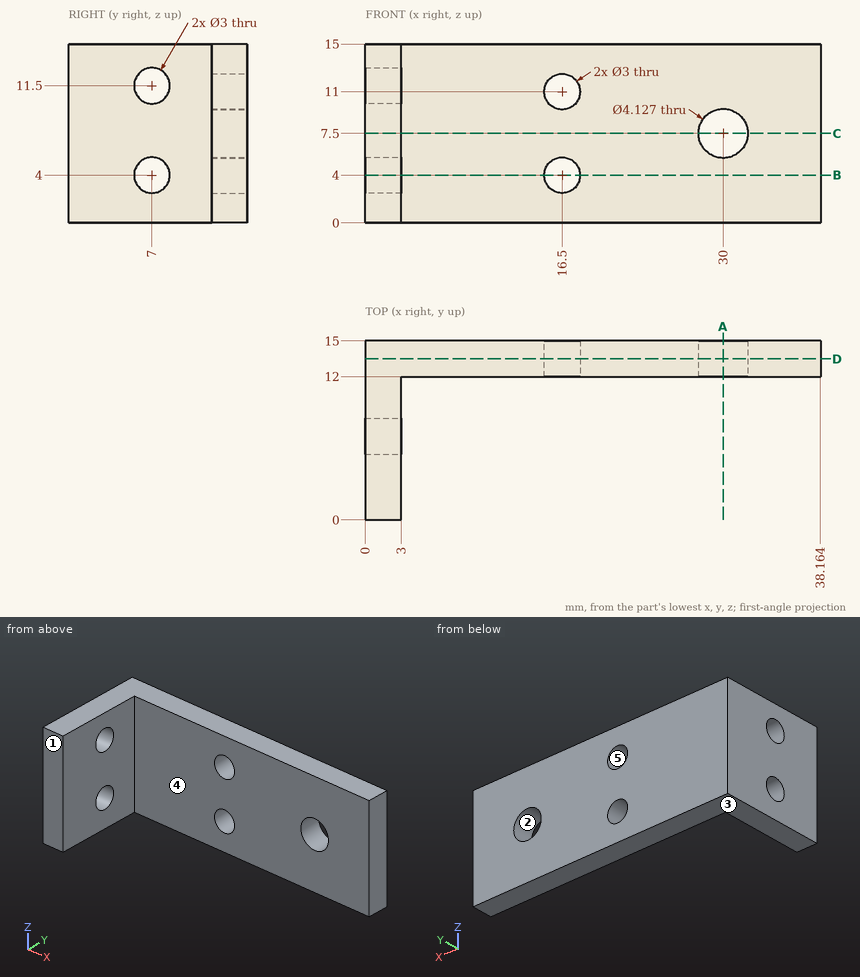
For this review, use the dimensioned drawing (mm, ordinates from the lowest corner) and the shaded views. A direction names the side the tool comes from. Round coordinates to 2 decimals unless told otherwise and drop trailing zeros. Write each loop counter-clockwise with the first axis right and the second up, starting at its lowest first coordinate (ties: lowest second). Pieces come first, ordered by that corner, then holes. Notation, with made-up numbers: (-37.5, 76.5) - (13.5, 76.5) arc R21 ccw to (13.5, 94.5) - close; hole circle Ø4 at (24.25, 59). An arc over 180 degrees is marked (long way). Answer as a JSON object with one key per item and string values.
1. For pin 1 Ø4 at (x, z) = (16.5, 11) entering from -Y; pin 2 Ø8 at (y, z) = (10.5, 3) entering from -X; pin 3 Ø8 at (y, z) = (2, 2) entering from +X, all flat-tipped, find the tip position at first contact; note any pin that passes through.
Response values:
{"pin 1": "stops at y = 12", "pin 2": "stops at x = 0", "pin 3": "stops at x = 3"}
2. We need section B-B on z = 4. Give the boundary of the cut face in (x, y).
Response values:
{"outline": "(0, 0) - (3, 0) - (3, 5.5) - (0, 5.5) - close; (0, 8.5) - (3, 8.5) - (3, 12) - (15, 12) - (15, 15) - (0, 15) - close; (18, 12) - (38.16, 12) - (38.16, 15) - (18, 15) - close"}
3. Tool access review of the marked faces 4 and 5: name each direction out of +Z, -Z, +X, -X, +Y, -Y from which nothing blocks a thin tool from reaching the whole face with its end or side.
Response values:
{"face 4": "+Z, -Z, +X, -Y", "face 5": "+Y, -Y"}
4. Draft analysis for pull direction Z (two halves, no side actions). For the marked faces 1, 2 and 3, state which applies: +Z half, -Z half, draft (parallel to the pull), parting line (faces both ways), or undercut.
Response values:
{"face 1": "draft", "face 2": "undercut", "face 3": "-Z half"}
5. We need section D-D on y = 13.5. Give the boundary of the cut face in (x, z), then the cut area to 3 significant figures.
Response values:
{"outline": "(0, 0) - (38.16, 0) - (38.16, 15) - (0, 15) - close; hole circle Ø3 at (16.5, 4); hole circle Ø3 at (16.5, 11); hole circle Ø4.13 at (30, 7.5)", "area": "545 mm2"}
6. We need section A-A on x = 30. Give the boundary of the cut face in (y, z), then the cut area to 3 significant figures.
Response values:
{"outline": "(12, 0) - (15, 0) - (15, 5.44) - (12, 5.44) - close; (12, 9.56) - (15, 9.56) - (15, 15) - (12, 15) - close", "area": "32.6 mm2"}
7. To check wall thickness, follow line 1 along Z through (x, y) = (16.5, 14.1); line 2 along X through (y, z) = (13, 7.5); line 3 along X through (y, z) = (14.2, 4). State the ranges of each line that lie inside material, in increasing order.
Response values:
{"line 1": "z = 0 to 2.5, 5.5 to 9.5, 12.5 to 15", "line 2": "x = 0 to 27.94, 32.06 to 38.16", "line 3": "x = 0 to 15, 18 to 38.16"}
8. We need section C-C on z = 7.5. Give the boundary of the cut face in (x, y), then the cut area to 3 significant figures.
Response values:
{"outline": "(0, 0) - (3, 0) - (3, 12) - (27.94, 12) - (27.94, 15) - (0, 15) - close; (32.06, 12) - (38.16, 12) - (38.16, 15) - (32.06, 15) - close", "area": "138 mm2"}
